Read the model definition and answer for the solid it produces. Units are mm, in the model's axes. A direction names the side the tool comes from. Coordinates: 2 decimals unless noted, no trailing zeros. Write each loop counter-clockwise with the first axis right and the second up, starting at its lowest first coordinate (ties: lowest second). Pieces come first, ordered by that corner, then holes. Notation, with made-up numbers: (89, 67) -> (104, 67) arc R16 ccw to (104, 88) -> close; hole circle Ø8 at (-29.75, 7.5). An arc over 180 degrees is marked (long way). Write item = value, one per line. Start each with the question number.
1) Section B-B (x = 12) is taken. Determine the outline of the cut face in (y, z).
2) Section A-A (x = -12) is taken. Determine the outline of the cut face in (y, z).
3) A tool of negligible diameter and unlimited length cuts with its end or side. For faces 1 (the face through (-10.652, -15, -42)), 2 (the face through (-16.902, -15, -1)), 3 (the face through (10.652, -15, -42)), 4 (the face through (-10.602, -15, 42)), 5 (the face through (15, -15, 37.752)), from which of +Z, -Z, +X, -X, +Y, -Y can it reach the whole face along a straight path? Write none if from no direction.
4) Find the intervals of material crossed by line 1 along Z through (x, y) = (-15, -14.45); line 2 along Z through (x, y) = (14, -14.35); line 3 along X through (y, z) = (-14, 40), in increasing order. Write a range as from..to.
5) Flat-ended cylindrical pins translate along their axes: pin 1 Ø0.8 at (y, z) = (-14.5, -42.5) entering from -X; pin 2 Ø0.8 at (x, y) = (-15, -14.5) entering from +Z; pin 3 Ø0.8 at (x, y) = (15, -14.5) entering from +Z. Find the tip coordinate at first contact, or state that the pin passes through.
from build123d import *

# Parameters (mm, degrees)
EFFECTSBOARD_DEPTH = 1.57


with BuildPart() as part:
    # Sketch2 → EffectsBoard (new body)
    with BuildSketch(Plane(origin=(0, -15.44984767, 0), x_dir=(-1, 0, 0), z_dir=(0, -1, 0))):
        with BuildLine():
            Line((9.702810165, -43.95246749), (-9.802810165, -43.95246749))
            add(Edge.make_bspline(
                [(-9.802810165, -43.95246749), (-9.915209225, -43.95246749), (-10.13503537, -43.913811014), (-10.458796653, -43.708796653), (-10.663811014, -43.38503537), (-10.70246749, -43.165209225), (-10.70246749, -43.052810165)],
                knots=[0, 0, 0, 0, 0.25, 0.5, 0.75, 1, 1, 1, 1], degree=3))
            Line((-10.70246749, -43.052810165), (-10.70246749, -41.3))
            ThreePointArc((-10.70246749, -41.3), (-11.741515706, -38.791515706), (-14.25, -37.75246749))
            Line((-14.25, -37.75246749), (-16.002810165, -37.75246749))
            add(Edge.make_bspline(
                [(-16.002810165, -37.75246749), (-16.115209225, -37.75246749), (-16.33503537, -37.713811014), (-16.658796653, -37.508796653), (-16.863811014, -37.18503537), (-16.90246749, -36.965209225), (-16.90246749, -36.852810165)],
                knots=[0, 0, 0, 0, 0.25, 0.5, 0.75, 1, 1, 1, 1], degree=3))
            Line((-16.90246749, -36.852810165), (-16.90246749, 36.802810165))
            add(Edge.make_bspline(
                [(-16.90246749, 36.802810165), (-16.90246749, 36.915209225), (-16.863811014, 37.13503537), (-16.658796653, 37.458796653), (-16.33503537, 37.663811014), (-16.115209225, 37.70246749), (-16.002810165, 37.70246749)],
                knots=[0, 0, 0, 0, 0.25, 0.5, 0.75, 1, 1, 1, 1], degree=3))
            Line((-16.002810165, 37.70246749), (-14.25, 37.70246749))
            ThreePointArc((-14.25, 37.70246749), (-11.706160367, 38.756160367), (-10.65246749, 41.3))
            Line((-10.65246749, 41.3), (-10.65246749, 43.052810165))
            add(Edge.make_bspline(
                [(-10.65246749, 43.052810165), (-10.65246749, 43.165209225), (-10.613811014, 43.38503537), (-10.408796653, 43.708796653), (-10.08503537, 43.913811014), (-9.865209225, 43.95246749), (-9.752810165, 43.95246749)],
                knots=[0, 0, 0, 0, 0.25, 0.5, 0.75, 1, 1, 1, 1], degree=3))
            Line((-9.752810165, 43.95246749), (9.752810165, 43.95246749))
            add(Edge.make_bspline(
                [(9.752810165, 43.95246749), (9.865209225, 43.95246749), (10.08503537, 43.913811014), (10.408796653, 43.708796653), (10.613811014, 43.38503537), (10.65246749, 43.165209225), (10.65246749, 43.052810165)],
                knots=[0, 0, 0, 0, 0.25, 0.5, 0.75, 1, 1, 1, 1], degree=3))
            Line((10.65246749, 43.052810165), (10.65246749, 41.3))
            ThreePointArc((10.65246749, 41.3), (11.706160367, 38.756160367), (14.25, 37.70246749))
            Line((14.25, 37.70246749), (16.002810165, 37.70246749))
            add(Edge.make_bspline(
                [(16.002810165, 37.70246749), (16.115209225, 37.70246749), (16.33503537, 37.663811014), (16.658796653, 37.458796653), (16.863811014, 37.13503537), (16.90246749, 36.915209225), (16.90246749, 36.802810165)],
                knots=[0, 0, 0, 0, 0.25, 0.5, 0.75, 1, 1, 1, 1], degree=3))
            Line((16.90246749, 36.802810165), (16.90246749, -36.752810165))
            add(Edge.make_bspline(
                [(16.90246749, -36.752810165), (16.90246749, -36.865209225), (16.863811014, -37.08503537), (16.658796653, -37.408796653), (16.33503537, -37.613811014), (16.115209225, -37.65246749), (16.002810165, -37.65246749)],
                knots=[0, 0, 0, 0, 0.25, 0.5, 0.75, 1, 1, 1, 1], degree=3))
            Line((16.002810165, -37.65246749), (14.25, -37.65246749))
            ThreePointArc((14.25, -37.65246749), (11.670805028, -38.720805028), (10.60246749, -41.3))
            Line((10.60246749, -41.3), (10.60246749, -43.052810165))
            add(Edge.make_bspline(
                [(10.60246749, -43.052810165), (10.60246749, -43.165209225), (10.563811014, -43.38503537), (10.358796653, -43.708796653), (10.03503537, -43.913811014), (9.815209225, -43.95246749), (9.702810165, -43.95246749)],
                knots=[0, 0, 0, 0, 0.25, 0.5, 0.75, 1, 1, 1, 1], degree=3))
        make_face()
    extrude(amount=-EFFECTSBOARD_DEPTH)


solid = part.part
Answer key:
q1.outline = (-15.45, -38.49) -> (-13.88, -38.49) -> (-13.88, 38.56) -> (-15.45, 38.56) -> close
q2.outline = (-15.45, -38.49) -> (-13.88, -38.49) -> (-13.88, 38.43) -> (-15.45, 38.43) -> close
q3.face_1 = -Z, -X, +Y, -Y
q3.face_2 = +Z, -Z, -X, +Y, -Y
q3.face_3 = -Z, +X, +Y, -Y
q3.face_4 = +Z, -X, +Y, -Y
q3.face_5 = +Z, +X, +Y, -Y
q4.line_1 = -37.7..37.65
q4.line_2 = -37.71..37.76
q4.line_3 = -10.84..10.95
q5.pin_1 = -10.65
q5.pin_2 = 37.65
q5.pin_3 = 37.75
